Could you check a few things on this model? Use its own coordinates, in mm. A direction names the side the tool comes from. Give positions to 0.01 mm unless a question says otherwise; leave off trailing zeros. Write each loop counter-clockwise with the first axis right and the second up, starting at its lowest first coordinate (ties: lowest second). Pieces come first, ordered by that corner, then holes. Notation, with made-up numbers: M -6,31 L -2,31 A21 ccw -2,49 Z; hole C 21.5,37.25 d1. An arc over 180 degrees is marked long. One line per item, written item: value.
```python
from build123d import *

# Parameters (mm, degrees)
SKETCH1_W           = 180
SKETCH1_H           = 180
SKETCH1_R           = 1.5
BOSS_EXTRUDE1_DEPTH = 3
SKETCH2_R           = 1.5
CUT_EXTRUDE1_DEPTH  = 4
SKETCH3_R           = 5
BOSS_EXTRUDE2_DEPTH = 350


with BuildPart() as part:
    # Sketch1 → Boss-Extrude1 (new body)
    with BuildSketch(Plane(origin=(0, 0, 0), x_dir=(1, 0, 0), z_dir=(0, 1, 0))):
        with Locations((-90, 90)):
            Rectangle(SKETCH1_W, SKETCH1_H)
        with Locations((-90, 90)):
            Circle(SKETCH1_R, mode=Mode.SUBTRACT)
        with Locations((-58, 90)):
            Circle(SKETCH1_R, mode=Mode.SUBTRACT)
        with Locations((-122, 90)):
            Circle(SKETCH1_R, mode=Mode.SUBTRACT)
        with Locations((-90, 122)):
            Circle(SKETCH1_R, mode=Mode.SUBTRACT)
        with Locations((-90, 58)):
            Circle(SKETCH1_R, mode=Mode.SUBTRACT)
    extrude(amount=BOSS_EXTRUDE1_DEPTH)

    # Sketch2 → Cut-Extrude1 (cut, through all)
    with BuildSketch(Plane(origin=(0, 3, 0), x_dir=(1, 0, 0), z_dir=(0, 1, 0))):
        with Locations((-147.18268, 90)):
            Circle(SKETCH2_R)
        with Locations((-129.18268, 90)):
            Circle(SKETCH2_R)
    extrude(amount=-CUT_EXTRUDE1_DEPTH, mode=Mode.SUBTRACT)

    # Sketch3 → Boss-Extrude2 (add)
    with BuildSketch(Plane.XZ):
        with Locations((-172, -8)):
            Circle(SKETCH3_R)
        with Locations((-8, -8)):
            Circle(SKETCH3_R)
        with Locations((-8, -172)):
            Circle(SKETCH3_R)
        with Locations((-172, -172)):
            Circle(SKETCH3_R)
    extrude(amount=BOSS_EXTRUDE2_DEPTH)


solid = part.part
```
1) If we section it at A-A, the plane z = -8: Write out the boundary of the cut face in (x, y).
Outcome:
outline: M -180,0 L -177,0 L -177,-350 L -167,-350 L -167,0 L -13,0 L -13,-350 L -3,-350 L -3,0 L 0,0 L 0,3 L -180,3 Z
2) Please list where these lines run through material, in increasing order: L1, parallel to Z at x = -171.5, y = -240.5; L2, parallel to Y at x = -144, z = -142.5; L3, parallel to Z at x = -122, y = 1.45. Write a range as from..to.
Outcome:
L1: z = -176.97..-167.03, -12.97..-3.03
L2: y = 0..3
L3: z = -180..-91.5, -88.5..0
3) I'm going to push flat-ended pins straight in: pin 1 (3.5 mm diameter, centred on x = -122, z = -90, fed in from -Y); pin 2 (2.5 mm diameter, centred on x = -90, z = -90, fed in from +Y). Where does each tip first touch, or does it pass through?
Outcome:
pin 1: stops at y = 0
pin 2: passes through
4) On a 3-axis mill with a long thin cutter (end or side, diameter ignored), from which of +Z, -Z, +X, -X, +Y, -Y can I reach the whole of each face in a straight line? I mean faces 1 (the face through (-172.651, -172.55, -167.043)), 2 (the face through (-91.3, 3, -91.3)). Say none if no direction works.
Outcome:
face 1: -Y
face 2: +Z, -Z, +X, -X, +Y
5) If we section it at D-D, the plane z = -117: Write out the boundary of the cut face in (x, y), then the cut area to 3 significant figures.
Outcome:
outline: M -180,0 L 0,0 L 0,3 L -180,3 Z
area: 540 mm^2
6) If we section it at C-C, the plane x = -8: Write out the boundary of the cut face in (y, z), then the cut area to 3 significant figures.
Outcome:
outline: M -350,-177 L 0,-177 L 0,-180 L 3,-180 L 3,0 L 0,0 L 0,-3 L -350,-3 L -350,-13 L 0,-13 L 0,-167 L -350,-167 Z
area: 7,540 mm^2
7) If we section it at B-B, the plane y = -219.5: Write out the boundary of the cut face in (x, z).
Outcome:
outline: C -172,-172 d10; C -172,-8 d10; C -8,-172 d10; C -8,-8 d10
8) We'd pull the mould along Z, two halves only. Please class faces 3 (the face through (-177, -173, -8)), 4 (the face through (-8, -350, -172)), 5 (the face through (-8.651, -172.55, -167.043)): pulls with the +Z half, pulls with the -Z half, needs draft (parallel to the pull), parting line crosses it, or undercut.
Outcome:
face 3: undercut
face 4: needs draft
face 5: undercut
